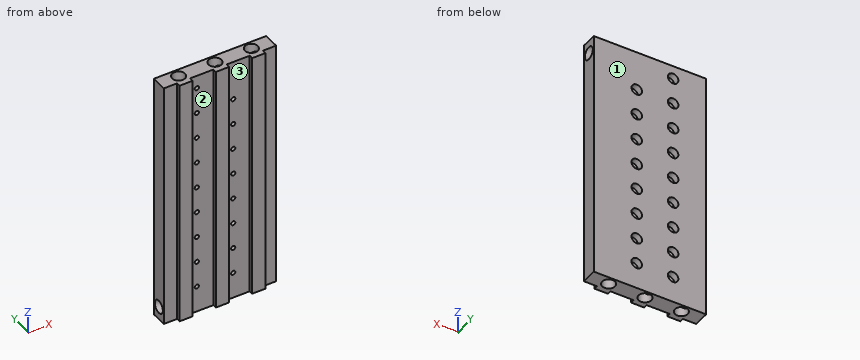
```python
from build123d import *

# Parameters (mm, degrees)
SKETCH1_R           = 4.864
BOSS_EXTRUDE1_DEPTH = 190
SKETCH2_R           = 4.864
CUT_EXTRUDE1_DEPTH  = 40
SKETCH5_R           = 4.864
CUT_EXTRUDE3_DEPTH  = 40
SKETCH6_R           = 1.6
CUT_EXTRUDE4_DEPTH  = 209.686367547
SKETCH7_R           = 4
CUT_EXTRUDE5_DEPTH  = 5


with BuildPart() as part:
    # Sketch1 → Boss-Extrude1 (new body)
    with BuildSketch(Plane.XY):
        Polygon((37.5, 0), (37.5, -3), (47.5, -3), (47.5, 0), (65, 0), (65, -3), (75, -3), (75, 0), (85, 0), (85, 12), (0, 12), (0, 0), (10, 0), (10, -3), (20, -3), (20, 0), align=None)
        with Locations((15, 6)):
            Circle(SKETCH1_R, mode=Mode.SUBTRACT)
        with Locations((42.5, 6)):
            Circle(SKETCH1_R, mode=Mode.SUBTRACT)
        with Locations((70, 6)):
            Circle(SKETCH1_R, mode=Mode.SUBTRACT)
    extrude(amount=BOSS_EXTRUDE1_DEPTH)

    # Sketch2 → Cut-Extrude1 (cut)
    with BuildSketch(Plane(origin=(85, 0, 0), x_dir=(0, 0, -1), z_dir=(1, 0, 0))):
        with Locations((-180, 6)):
            Circle(SKETCH2_R)
    extrude(amount=-CUT_EXTRUDE1_DEPTH, mode=Mode.SUBTRACT)

    # Sketch5 → Cut-Extrude3 (cut)
    with BuildSketch(Plane.ZY):
        with Locations(Location((10, 6, 0), (0, 0, 59.070681313))):
            Circle(SKETCH5_R)
    extrude(amount=-CUT_EXTRUDE3_DEPTH, mode=Mode.SUBTRACT)

    # Sketch6 → Cut-Extrude4 (cut, through all)
    with BuildSketch(Plane(origin=(0, 12, 0), x_dir=(1, 0, 0), z_dir=(0, 1, 0))):
        with Locations(Location((25, -180, 0), (0, 0, 270))):
            Circle(SKETCH6_R)
        with Locations(Location((52.5, -160, 0), (0, 0, 270))):
            Circle(SKETCH6_R)
        with Locations(Location((52.5, -140, 0), (0, 0, 270))):
            Circle(SKETCH6_R)
        with Locations(Location((52.5, -120, 0), (0, 0, 270))):
            Circle(SKETCH6_R)
        with Locations(Location((52.5, -100, 0), (0, 0, 270))):
            Circle(SKETCH6_R)
        with Locations(Location((52.5, -80, 0), (0, 0, 270))):
            Circle(SKETCH6_R)
        with Locations(Location((52.5, -60, 0), (0, 0, 270))):
            Circle(SKETCH6_R)
        with Locations(Location((52.5, -40, 0), (0, 0, 270))):
            Circle(SKETCH6_R)
        with Locations(Location((52.5, -20, 0), (0, 0, 270))):
            Circle(SKETCH6_R)
        with Locations(Location((25, -160, 0), (0, 0, 270))):
            Circle(SKETCH6_R)
        with Locations(Location((25, -140, 0), (0, 0, 270))):
            Circle(SKETCH6_R)
        with Locations(Location((25, -120, 0), (0, 0, 270))):
            Circle(SKETCH6_R)
        with Locations(Location((25, -100, 0), (0, 0, 270))):
            Circle(SKETCH6_R)
        with Locations(Location((25, -80, 0), (0, 0, 270))):
            Circle(SKETCH6_R)
        with Locations(Location((25, -60, 0), (0, 0, 270))):
            Circle(SKETCH6_R)
        with Locations(Location((25, -40, 0), (0, 0, 270))):
            Circle(SKETCH6_R)
        with Locations(Location((25, -20, 0), (0, 0, 270))):
            Circle(SKETCH6_R)
    extrude(amount=-CUT_EXTRUDE4_DEPTH, mode=Mode.SUBTRACT)

    # Sketch7 → Cut-Extrude5 (cut)
    with BuildSketch(Plane(origin=(0, 12, 0), x_dir=(1, 0, 0), z_dir=(0, 1, 0))):
        with Locations(Location((25, -180, 0), (0, 0, 270))):
            Circle(SKETCH7_R)
        with Locations(Location((52.5, -160, 0), (0, 0, 270))):
            Circle(SKETCH7_R)
        with Locations(Location((52.5, -140, 0), (0, 0, 270))):
            Circle(SKETCH7_R)
        with Locations(Location((52.5, -120, 0), (0, 0, 270))):
            Circle(SKETCH7_R)
        with Locations(Location((52.5, -100, 0), (0, 0, 270))):
            Circle(SKETCH7_R)
        with Locations(Location((52.5, -80, 0), (0, 0, 270))):
            Circle(SKETCH7_R)
        with Locations(Location((52.5, -60, 0), (0, 0, 270))):
            Circle(SKETCH7_R)
        with Locations(Location((52.5, -40, 0), (0, 0, 270))):
            Circle(SKETCH7_R)
        with Locations(Location((52.5, -20, 0), (0, 0, 270))):
            Circle(SKETCH7_R)
        with Locations(Location((25, -160, 0), (0, 0, 270))):
            Circle(SKETCH7_R)
        with Locations(Location((25, -140, 0), (0, 0, 270))):
            Circle(SKETCH7_R)
        with Locations(Location((25, -120, 0), (0, 0, 270))):
            Circle(SKETCH7_R)
        with Locations(Location((25, -100, 0), (0, 0, 270))):
            Circle(SKETCH7_R)
        with Locations(Location((25, -80, 0), (0, 0, 270))):
            Circle(SKETCH7_R)
        with Locations(Location((25, -60, 0), (0, 0, 270))):
            Circle(SKETCH7_R)
        with Locations(Location((25, -40, 0), (0, 0, 270))):
            Circle(SKETCH7_R)
        with Locations(Location((25, -20, 0), (0, 0, 270))):
            Circle(SKETCH7_R)
    extrude(amount=-CUT_EXTRUDE5_DEPTH, mode=Mode.SUBTRACT)


solid = part.part
```
Check sheet for the modelled part. Datum: model origin and axes. Units: mm. Face numbers are marked on the shaded views. Round coordinates to 2 decimals unless told otherwise and drop trailing zeros. Loops run counter-clockwise (first coordinate to the right, second up) from the corner with the lowest first, then second, coordinate; pieces in that order, holes last. Notation, with made-up numbers: (-8.75, 43) -> (48.25, 43) arc R29 cw to (48.25, 64) -> close; hole circle Ø1 at (24, -13.75). An arc over 180 degrees is marked (long way). Write item = value, one per line. Start each with the question number.
1) Thickness scan on probe 1 along X at (y, z) = (-2.5, 140); probe 2 along Z at (x, y) = (80.5, 6); probe 3 along X at (y, z) = (5.25, 61). Record the ranges inside material, lowest first.
2) Release check for a two-part mould opening along X. For the marked faces 1, 2 and 3 record: released by +X, released by -X, zero draft, split by the parting line, or undercut.
3) Sectioned sample at C-C, the plane x = 67.5. Record the cut outline in (y, z).
4) Sectioned sample at B-B, the plane z = 149.5. Record the cut outline in (x, y), plus the area to 3 significant figures.
5) Sectioned sample at A-A, the plane x = 42.5. Record the cut outline in (y, z), plus the area to 3 significant figures.
6) Gauge pin test, flat ends, axial feed: pin 1 Ø3.5 at (y, z) = (-2, 103.5) entering from -X; pin 2 Ø6.5 at (x, z) = (25, 80) entering from -Y; pin 3 Ø2.5 at (x, z) = (26.5, 121) entering from +Y. Record the tip position at first contact, or that the pin passes through.
Results are:
q1.probe_1 = 10 to 20, 37.5 to 47.5, 65 to 75
q1.probe_2 = 0 to 175.14, 184.86 to 190
q1.probe_3 = 0 to 10.19, 19.81 to 23.75, 26.25 to 37.69, 47.31 to 51.25, 53.75 to 65.19, 74.81 to 85
q2.face_1 = zero draft
q2.face_2 = undercut
q2.face_3 = undercut
q3.outline = (-3, 0) -> (1.83, 0) -> (1.83, 177.5) arc R4.86 cw to (1.83, 182.5) -> (1.83, 190) -> (-3, 190) -> close; (10.17, 0) -> (12, 0) -> (12, 190) -> (10.17, 190) -> (10.17, 182.5) arc R4.86 cw to (10.17, 177.5) -> close
q4.outline = (0, 0) -> (10, 0) -> (10, -3) -> (20, -3) -> (20, 0) -> (37.5, 0) -> (37.5, -3) -> (47.5, -3) -> (47.5, 0) -> (65, 0) -> (65, -3) -> (75, -3) -> (75, 0) -> (85, 0) -> (85, 12) -> (0, 12) -> close; hole circle Ø9.73 at (15, 6); hole circle Ø9.73 at (42.5, 6); hole circle Ø9.73 at (70, 6)
q4.area = 887 mm^2
q5.outline = (-3, 0) -> (1.14, 0) -> (1.14, 190) -> (-3, 190) -> close; (10.86, 0) -> (12, 0) -> (12, 190) -> (10.86, 190) -> close
q5.area = 1,000 mm^2
q6.pin_1 = 10
q6.pin_2 = 0
q6.pin_3 = 7
